For this review, take the finished solid that the model builds, in its own axes (mm). A direction names the side the tool comes from. Coordinates: 2 decimals unless noted, no trailing zeros. Write each loop counter-clockwise with the first axis right and the second up, starting at its lowest first coordinate (ties: lowest second). Pieces come first, ordered by that corner, then holes. Notation, with made-up numbers: M 57,50.5 L 78,50.5 A13 cw 78,66.5 Z; hole C -29,69 d5. An arc over 180 degrees is marked long. One line per question, with ' | ' between items.
Autodesk Inventor part; units mm, degrees
ref_plane "XY Plane" through (0, 0, 0) normal (0, 0, 1) x (1, 0, 0)
sketch "Эскиз1" plane through (0, 0, 0) normal (0, 1, 0) x (-1, 0, 0)
  line L0 (5.5, 5) -> (-5.5, 5)
  line L1 (-5.5, 5) -> (-5.5, -5)
  line L2 (-5.5, -5) -> (5.5, -5)
  line L3 (5.5, -5) -> (5.5, 5)
  line L4 (5.5, 5) -> (-5.5, -5) construction
  line L5 (-5.5, 5) -> (5.5, -5) construction
  point P0 (0, 0)
  dimension "d0" = 11
  dimension "d1" = 10
ref_plane "РабПлоскость1" through (0, 2.5, 0) normal (0, 1, 0) x (1, 0, 0)
sketch "Эскиз3" plane through (0, 2.5, 0) normal (0, 1, 0) x (1, 0, 0)
  arc A0 (-5.15, 5) -> (-4.9, 5.25) centre (-5.15, 5.25) ccw
  line L0 (-4.9, 5.8) -> (-4.9, 5.25)
  line L1 (-4.35, 5.8) -> (-4.9, 5.8)
  arc A1 (-4.35, 5.8) -> (-4.1, 6.05) centre (-4.35, 6.05) ccw
  line L2 (-4.1, 6.95) -> (-4.1, 6.05)
  arc A2 (-4.1, 6.95) -> (-4.35, 7.2) centre (-4.35, 6.95) ccw
  line L3 (-5.439, 7.2) -> (-4.35, 7.2)
  arc A3 (-5.439, 7.2) -> (-5.6666, 7.0535) centre (-5.439, 6.95) ccw
  line L4 (-6.0258, 6.2631) -> (-5.6666, 7.0535)
  arc A4 (-6.2783, 6.1178) -> (-6.0258, 6.2631) centre (-6.2534, 6.3666) ccw
  line L5 (-7.8749, 6.2775) -> (-6.2783, 6.1178)
  arc A5 (-8.1, 6.5262) -> (-7.8749, 6.2775) centre (-7.85, 6.5262) ccw
  line L6 (-8.1, 10.8115) -> (-8.1, 6.5262)
  arc A6 (-7.8803, 11.3419) -> (-8.1, 10.8115) centre (-7.35, 10.8115) ccw
  arc A7 (8.1, 10.8115) -> (7.8803, 11.3419) centre (7.35, 10.8115) ccw
  line L7 (8.1, 6.5262) -> (8.1, 10.8115)
  arc A8 (7.8749, 6.2775) -> (8.1, 6.5262) centre (7.85, 6.5262) ccw
  line L8 (6.2783, 6.1178) -> (7.8749, 6.2775)
  arc A9 (6.0258, 6.2631) -> (6.2783, 6.1178) centre (6.2534, 6.3666) ccw
  line L9 (5.6666, 7.0535) -> (6.0258, 6.2631)
  arc A10 (5.6666, 7.0535) -> (5.439, 7.2) centre (5.439, 6.95) ccw
  line L10 (4.35, 7.2) -> (5.439, 7.2)
  arc A11 (4.35, 7.2) -> (4.1, 6.95) centre (4.35, 6.95) ccw
  line L11 (4.1, 6.05) -> (4.1, 6.95)
  arc A12 (4.1, 6.05) -> (4.35, 5.8) centre (4.35, 6.05) ccw
  line L12 (4.9, 5.8) -> (4.35, 5.8)
  line L13 (4.9, 5.25) -> (4.9, 5.8)
  arc A13 (4.9, 5.25) -> (5.15, 5) centre (5.15, 5.25) ccw
  line L14 (7.8803, 11.3419) -> (6.4419, 12.7803)
  arc A14 (6.4419, 12.7803) -> (5.9115, 13) centre (5.9115, 12.25) ccw
  line L15 (5.9115, 13) -> (0.4906, 13)
  line L16 (-0.4906, 13) -> (-5.9115, 13)
  arc A15 (-5.9115, 13) -> (-6.4419, 12.7803) centre (-5.9115, 12.25) ccw
  line L17 (-6.4419, 12.7803) -> (-7.8803, 11.3419)
  line L18 (0.4906, 13) -> (-0.4906, 13)
  line L19 (-3.7, 6.05) -> (-3.7, 6.95)
  arc A16 (-3.7, 6.95) -> (-4.35, 7.6) centre (-4.35, 6.95) ccw
  line L20 (-4.35, 7.6) -> (-5.439, 7.6)
  arc A17 (-5.439, 7.6) -> (-6.0308, 7.219) centre (-5.439, 6.95) ccw
  line L21 (-6.0308, 7.219) -> (-6.3455, 6.5265)
  line L22 (-6.3455, 6.5265) -> (-7.7, 6.662)
  line L23 (-7.7, 6.662) -> (-7.7, 10.8115)
  arc A18 (-7.5975, 11.059) -> (-7.7, 10.8115) centre (-7.35, 10.8115) ccw
  line L24 (-7.5975, 11.059) -> (-6.159, 12.4975)
  arc A19 (-5.9115, 12.6) -> (-6.159, 12.4975) centre (-5.9115, 12.25) ccw
  line L25 (-5.9115, 12.6) -> (-0.4906, 12.6)
  line L26 (-0.4906, 12.6) -> (0.4906, 12.6)
  line L27 (0.4906, 12.6) -> (5.9115, 12.6)
  arc A20 (6.159, 12.4975) -> (5.9115, 12.6) centre (5.9115, 12.25) ccw
  line L28 (6.159, 12.4975) -> (7.5975, 11.059)
  arc A21 (7.7, 10.8115) -> (7.5975, 11.059) centre (7.35, 10.8115) ccw
  line L29 (7.7, 10.8115) -> (7.7, 6.662)
  line L30 (7.7, 6.662) -> (6.3455, 6.5265)
  line L31 (6.3455, 6.5265) -> (6.0308, 7.219)
  arc A22 (6.0308, 7.219) -> (5.439, 7.6) centre (5.439, 6.95) ccw
  line L32 (5.439, 7.6) -> (4.35, 7.6)
  arc A23 (4.35, 7.6) -> (3.7, 6.95) centre (4.35, 6.95) ccw
  line L33 (3.7, 6.95) -> (3.7, 6.1534)
  line L34 (-3.7, 5) -> (3.7, 5)
  line L35 (3.7, 5) -> (3.7, 6.1534)
  line L36 (-3.7, 6.05) -> (-3.7, 5)
  point P0 (0, 0)
  point P1 (-4.9967, 19.8192)
  dimension "d6" = 0.4
  dimension "d11" = 1.95
extrude "Выдавливание3" add sketch "Эскиз3" along normal mid plane 15
sketch "Эскиз4" plane through (5.9115, 10, -12.6) normal (0, 0, -1) x (-1, 0, 0)
  line L0 (2.4115, -5.4793) -> (5.9115, -3.4585)
  line L1 (5.9115, -3.4585) -> (9.4115, -5.4793)
  line L2 (9.4115, -5.4793) -> (9.4115, -9.5207)
  line L3 (9.4115, -9.5207) -> (5.9115, -11.5415)
  line L4 (5.9115, -11.5415) -> (2.4115, -9.5207)
  line L5 (2.4115, -9.5207) -> (2.4115, -5.4793)
  line L6 (11.823, -15) -> (0, -15)
  line L7 (-4.8685, -7.5) -> (16.6915, -7.5) construction
  line L8 (5.9115, -18) -> (5.9115, 3) construction
  point P0 (5.9115, -10)
  point P1 (5.9115, -7.5)
  dimension "d13" = 7
extrude "Выдавливание4" cut sketch "Эскиз4" against normal blind 3.2
sketch "Эскиз5" plane through (5.9115, 10, -9.4) normal (0, 0, -1) x (-1, 0, 0)
  circle A0 centre (5.9115, -7.5) radius 2.1
  line L0 (-4.8685, -7.5) -> (16.6915, -7.5) construction
  line L1 (5.9115, -18) -> (5.9115, 3) construction
  point P0 (5.9115, -10)
  dimension "d16" = 4.2
extrude "Выдавливание5" cut sketch "Эскиз5" against normal up to next
fillet "Сопряжение2" radius 1 4 edges at (-3.7, 2.5, -5) (3.7, 2.5, -5) (-7.7, 2.5, -6.662) (7.7, 2.5, -6.662)
properties part number "буль"
1) Insertion check: pin 1 Ø3 at (x, y) = (-5, 6) entering from +Z; pin 2 Ø0.9 at (x, y) = (-5, 3) entering from +Z; pin 3 Ø0.5 at (y, z) = (4, -6.5) entering from +X; pin 4 Ø7.5 at (x, y) = (1, 2.5) entering from -Z. Each pin has a flat end and moves straight along its axis. Give the tip position at first contact, or say it passes through.
Responses:
pin 1: z = -5.4 | pin 2: z = -7.6 | pin 3: x = 7.28 | pin 4: z = -12.6
2) We need section A-A on x = -0.5. State the section outline as (y, z) points.
Responses:
outline: M -5,-12.6 L -1.25,-12.6 L -1.25,-9.4 L 0.46,-9.4 L 0.46,-5 L -5,-5 Z; M 4.54,-9.4 L 6.25,-9.4 L 6.25,-12.6 L 10,-12.6 L 10,-5 L 4.54,-5 Z
3) The part is to be moulded in two halves that separate along Y. For faces 4 (the flat face through (2, 1, -9.4)), 5 (the flat face through (0, 10, -9)), 6 (the cylindrical face through (3.399, 2.605, -5.285)), say which applies: +Y half, -Y half, draft (parallel to the pull), parting line (faces both ways), or undercut.
Responses:
face 4: undercut | face 5: +Y half | face 6: draft
4) Machinability: for faces 1 (the flat face through (3.7, 2.4, -6.5)), 2 (the flat face through (1.8, 5.5, -11)), 3 (the cylindrical face through (-3.415, 2.605, -5.301)), which of the approach directions +Z, -Z, +X, -X, +Y, -Y give a long, thin tool a straight path to every point of the face, cutting with its end or side? Answer none if there is none.
Responses:
face 1: +Z, +Y, -Y | face 2: -Z | face 3: +Z, -X, +Y, -Y
5) To check wall thickness, follow line 1 along Y through (x, z) = (0, -6.15); line 2 along X through (y, z) = (1, -9.75); line 3 along X through (y, z) = (-3.75, -7). State the ranges of each line that lie inside material, in increasing order. Write a range as [from, to].
Responses:
line 1: [-5, 0.4], [4.6, 10] | line 2: [-7.7, -3.5], [3.5, 7.7] | line 3: [-7.52, -6.13], [-3.7, 3.7], [6.13, 7.52]
6) We need section C-C on y = -2.5. State the section outline as (x, z) points.
Responses:
outline: M -7.7,-10.81 A0.35 ccw -7.6,-11.06 L -6.16,-12.5 A0.35 ccw -5.91,-12.6 L 5.91,-12.6 A0.35 ccw 6.16,-12.5 L 7.6,-11.06 A0.35 ccw 7.7,-10.81 L 7.7,-7.57 A1 ccw 6.8,-6.57 L 6.35,-6.53 L 6.03,-7.22 A0.65 cw 5.44,-7.6 L 4.35,-7.6 A0.65 cw 3.7,-6.95 L 3.7,-6 A1 ccw 2.7,-5 L -2.7,-5 A1 ccw -3.7,-6 L -3.7,-6.95 A0.65 cw -4.35,-7.6 L -5.44,-7.6 A0.65 cw -6.03,-7.22 L -6.35,-6.53 L -6.8,-6.57 A1 ccw -7.7,-7.57 Z
7) We need section D-D on z = -8.75. State the section outline as (x, y) points.
Responses:
outline: M -7.7,-5 L 7.7,-5 L 7.7,10 L -7.7,10 Z; hole C 0,2.5 d4.2
